Source: CAD feature listing. Evaluate the final solid. Frame: model axes, mm. A direction names the side the tool comes from. Give positions to 0.01 mm unless a question says otherwise; leave off trailing zeros. Loops run counter-clockwise (first coordinate to the right, second up) from the corner with the lowest first, then second, coordinate; pieces in that order, holes last. Notation, with made-up numbers: M 40,49.25 L 94,49.25 A17 ccw 94,58.25 Z; hole C 9,70.5 d9. An arc over 180 degrees is marked long. Answer in a Markdown table with one row per item.
```python
from build123d import *

# Parameters (mm, degrees)
SKETCH1_R           = 1.5
BOSS_EXTRUDE1_DEPTH = 2
FILLET1_R           = 3
FILLET2_R           = 3
SKETCH2_R           = 3
CUT_EXTRUDE1_DEPTH  = 58.905094767


with BuildPart() as part:
    # Sketch1 → Boss-Extrude1 (new body)
    with BuildSketch(Plane.XY):
        with BuildLine():
            Line((-18, 29.5), (-18, -33.5))
            Line((-18, -33.5), (18, -33.5))
            Line((18, -33.5), (18, 29.5))
            Line((18, 29.5), (18, 51))
            ThreePointArc((18, 51), (16.828427125, 53.828427125), (14, 55))
            Line((14, 55), (9, 55))
            Line((9, 55), (9, 44))
            ThreePointArc((9, 44), (0, 35), (-9, 44))
            Line((-9, 44), (-9, 55))
            Line((-9, 55), (-14, 55))
            ThreePointArc((-14, 55), (-16.828427125, 53.828427125), (-18, 51))
            Line((-18, 51), (-18, 29.5))
        make_face()
        with Locations((-14, -29.5)):
            Circle(SKETCH1_R, mode=Mode.SUBTRACT)
        with Locations((14, -29.5)):
            Circle(SKETCH1_R, mode=Mode.SUBTRACT)
        with Locations((-13, 52)):
            Circle(SKETCH1_R, mode=Mode.SUBTRACT)
        with Locations(Location((13, 52, 0), (0, 0, 180))):
            Circle(SKETCH1_R, mode=Mode.SUBTRACT)
    extrude(amount=BOSS_EXTRUDE1_DEPTH)

    # Fillet1
    fillet1_edges = [part.edges().sort_by_distance(p)[0] for p in [
        (18, -33.5, 1),
        (-18, -33.5, 1),
    ]]
    fillet(fillet1_edges, radius=FILLET1_R)

    # Fillet2
    fillet2_edges = [part.edges().sort_by_distance(p)[0] for p in [
        (-9, 55, 1),
        (9, 55, 1),
    ]]
    fillet(fillet2_edges, radius=FILLET2_R)

    # Sketch2 → Cut-Extrude1 (cut, through all)
    with BuildSketch(Plane.XY.offset(2)):
        with Locations((6, -17.75)):
            Circle(SKETCH2_R)
        with Locations(Location((-6, -17.75, 0), (0, 0, 180))):
            Circle(SKETCH2_R)
        with Locations(Location((-6, -5.75, 0), (0, 0, 180))):
            Circle(SKETCH2_R)
        with Locations((6, -5.75)):
            Circle(SKETCH2_R)
        with Locations(Location((-6, 6.25, 0), (0, 0, 180))):
            Circle(SKETCH2_R)
        with Locations((6, 6.25)):
            Circle(SKETCH2_R)
        with Locations(Location((-6, 18.25, 0), (0, 0, 180))):
            Circle(SKETCH2_R)
        with Locations((6, 18.25)):
            Circle(SKETCH2_R)
        with Locations(Location((-6, 30.25, 0), (0, 0, 180))):
            Circle(SKETCH2_R)
        with Locations((6, 30.25)):
            Circle(SKETCH2_R)
        with BuildLine():
            Line((-15.5, 1.75), (-15.5, -19.25))
            ThreePointArc((-15.5, -19.25), (-14, -20.75), (-12.5, -19.25))
            Line((-12.5, -19.25), (-12.5, 1.75))
            ThreePointArc((-12.5, 1.75), (-14, 3.25), (-15.5, 1.75))
        make_face()
        with BuildLine():
            Line((12.5, 1.75), (12.5, -19.25))
            ThreePointArc((12.5, -19.25), (14, -20.75), (15.5, -19.25))
            Line((15.5, -19.25), (15.5, 1.75))
            ThreePointArc((15.5, 1.75), (14, 3.25), (12.5, 1.75))
        make_face()
        with BuildLine():
            Line((-15.5, 31.75), (-15.5, 10.75))
            ThreePointArc((-15.5, 10.75), (-14, 9.25), (-12.5, 10.75))
            Line((-12.5, 10.75), (-12.5, 31.75))
            ThreePointArc((-12.5, 31.75), (-14, 33.25), (-15.5, 31.75))
        make_face()
        with BuildLine():
            Line((12.5, 31.75), (12.5, 10.75))
            ThreePointArc((12.5, 10.75), (14, 9.25), (15.5, 10.75))
            Line((15.5, 10.75), (15.5, 31.75))
            ThreePointArc((15.5, 31.75), (14, 33.25), (12.5, 31.75))
        make_face()
        with BuildLine():
            Line((-9, -29.5), (-9, -27.5))
            ThreePointArc((-9, -27.5), (-8, -26.5), (-7, -27.5))
            Line((-7, -27.5), (-7, -29.5))
            ThreePointArc((-7, -29.5), (-8, -30.5), (-9, -29.5))
        make_face()
        with BuildLine():
            Line((-5, -29.5), (-5, -27.5))
            ThreePointArc((-5, -27.5), (-4, -26.5), (-3, -27.5))
            Line((-3, -27.5), (-3, -29.5))
            ThreePointArc((-3, -29.5), (-4, -30.5), (-5, -29.5))
        make_face()
        with BuildLine():
            Line((-1, -29.5), (-1, -27.5))
            ThreePointArc((-1, -27.5), (0, -26.5), (1, -27.5))
            Line((1, -27.5), (1, -29.5))
            ThreePointArc((1, -29.5), (0, -30.5), (-1, -29.5))
        make_face()
        with BuildLine():
            Line((3, -29.5), (3, -27.5))
            ThreePointArc((3, -27.5), (4, -26.5), (5, -27.5))
            Line((5, -27.5), (5, -29.5))
            ThreePointArc((5, -29.5), (4, -30.5), (3, -29.5))
        make_face()
        with BuildLine():
            Line((7, -29.5), (7, -27.5))
            ThreePointArc((7, -27.5), (8, -26.5), (9, -27.5))
            Line((9, -27.5), (9, -29.5))
            ThreePointArc((9, -29.5), (8, -30.5), (7, -29.5))
        make_face()
        with BuildLine():
            Line((-16, 44.5), (-14, 44.5))
            ThreePointArc((-14, 44.5), (-13.5, 44), (-14, 43.5))
            Line((-14, 43.5), (-14.25, 43.5))
            Line((-14.25, 43.5), (-14.25, 39.5))
            Line((-14.25, 39.5), (-14, 39.5))
            ThreePointArc((-14, 39.5), (-13.5, 39), (-14, 38.5))
            Line((-14, 38.5), (-16, 38.5))
            ThreePointArc((-16, 38.5), (-16.5, 39), (-16, 39.5))
            Line((-16, 39.5), (-15.75, 39.5))
            Line((-15.75, 39.5), (-15.75, 43.5))
            Line((-15.75, 43.5), (-16, 43.5))
            ThreePointArc((-16, 43.5), (-16.5, 44), (-16, 44.5))
        make_face()
        with BuildLine():
            Line((14.25, 39.5), (14, 39.5))
            ThreePointArc((14, 39.5), (13.5, 39), (14, 38.5))
            Line((14, 38.5), (16, 38.5))
            ThreePointArc((16, 38.5), (16.5, 39), (16, 39.5))
            Line((16, 39.5), (15.75, 39.5))
            Line((15.75, 39.5), (15.75, 43.5))
            Line((15.75, 43.5), (16, 43.5))
            ThreePointArc((16, 43.5), (16.5, 44), (16, 44.5))
            Line((16, 44.5), (14, 44.5))
            ThreePointArc((14, 44.5), (13.5, 44), (14, 43.5))
            Line((14, 43.5), (14.25, 43.5))
            Line((14.25, 43.5), (14.25, 39.5))
        make_face()
    extrude(amount=-CUT_EXTRUDE1_DEPTH, mode=Mode.SUBTRACT)


solid = part.part
```
1) Section B-B, the plane x = 0. Return loops of the section in (y, z).
Reply:
| item | result |
|---|---|
| outline | M -33.5,0 L -30.5,0 L -30.5,2 L -33.5,2 Z; M -26.5,0 L 35,0 L 35,2 L -26.5,2 Z |
2) Section D-D, the plane y = 13. Return loops of the section in (x, z).
Reply:
| item | result |
|---|---|
| outline | M -18,0 L -15.5,0 L -15.5,2 L -18,2 Z; M -12.5,0 L 12.5,0 L 12.5,2 L -12.5,2 Z; M 15.5,0 L 18,0 L 18,2 L 15.5,2 Z |
3) Section A-A, the plane y = -17.75. Return loops of the section in (x, z), then the cut area to 3 significant figures.
Reply:
| item | result |
|---|---|
| outline | M -18,0 L -15.5,0 L -15.5,2 L -18,2 Z; M -12.5,0 L -9,0 L -9,2 L -12.5,2 Z; M -3,0 L 3,0 L 3,2 L -3,2 Z; M 9,0 L 12.5,0 L 12.5,2 L 9,2 Z; M 15.5,0 L 18,0 L 18,2 L 15.5,2 Z |
| area | 36.0 mm² |
4) Pull-direction query (Y, two-part tool) for faces 1 (the flat face through (0, 11, 2)), 2 (the cylindrical face through (17.1, -32.64, 1.01)), 3 (the cylindrical face through (4, -26.5, 1)); classes: released by +Y, released by -Y, zero draft, split by the parting line, or undercut.
Reply:
| item | result |
|---|---|
| face 1 | zero draft |
| face 2 | released by -Y |
| face 3 | undercut |
5) Pin query (flat end, axial travel): pin 1 Ø1 at (x, z) = (-15, 0.5) entering from +Y. Return the tip coordinate at first contact, or that it passes through.
Reply:
| item | result |
|---|---|
| pin 1 | stops at y = 54.97 |
6) Material intervals for L1, parallel to X at y = 26, z = 1; L2, parallel to X at y = 18.5, z = 1.65; L3, parallel to Y at x = 15, z = 1.3, sorted ascending.
Reply:
| item | result |
|---|---|
| L1 | x = -18 to -15.5, -12.5 to 12.5, 15.5 to 18 |
| L2 | x = -18 to -15.5, -12.5 to -8.99, -3.01 to 3.01, 8.99 to 12.5, 15.5 to 18 |
| L3 | y = -33.5 to -30.62, -28.38 to -20.37, 2.87 to 9.63, 32.87 to 38.5, 44.5 to 54.87 |
7) Set-up query: faces 4 (the flat face through (9, 48, 1)), 5 (the flat face through (14.25, 42, 1)), 6 (the cylindrical face through (16.859, 53.797, 0.986)). Return all of +Z, -Z, +X, -X, +Y, -Y with unobstructed straight access to the full face (end or side cutting, diameter ignored); none if empty.
Reply:
| item | result |
|---|---|
| face 4 | +Z, -Z, +Y |
| face 5 | +Z, -Z |
| face 6 | +Z, -Z, +X, +Y |
8) Section C-C, the plane y = 48. Return loops of the section in (x, z).
Reply:
| item | result |
|---|---|
| outline | M -18,0 L -9,0 L -9,2 L -18,2 Z; M 9,0 L 18,0 L 18,2 L 9,2 Z |
